Could you check a few things on this model? Use its own coordinates, in mm. A direction names the side the tool comes from. Round coordinates to 2 decimals unless told otherwise and drop trailing zeros. Loops run counter-clockwise (first coordinate to the right, second up) from the corner with the lowest first, then second, coordinate; pieces in that order, holes last. Notation, with made-up numbers: (10.5, 17.25) -> (17.5, 17.25) arc R23 cw to (17.5, 54.25) -> close; hole circle Ø8 at (74, 45.5). An arc over 180 degrees is marked (long way). One line per item, written item: value.
```python
from build123d import *

# Parameters (mm, degrees)
SKETCH1_R           = 28.575
SKETCH1_R_2         = 14.2875
SKETCH1_R_3         = 2.667
BOSS_EXTRUDE1_DEPTH = 6.35
BOSS_EXTRUDE2_DEPTH = 6.35
SKETCH3_W           = 25.4
SKETCH3_H           = 12.7
BOSS_EXTRUDE3_DEPTH = 6.35
CUT_EXTRUDE4_REACH  = 101.646
SKETCH4_R           = 4.7625
FILLET1_R           = 6.35
SKETCH5_W           = 86.18949407
SKETCH5_H           = 10.684979127
CUT_EXTRUDE5_DEPTH  = 100.646453148


with BuildPart() as part:
    # Sketch1 → Boss-Extrude1 (new body)
    with BuildSketch(Plane(origin=(0, 0, 0), x_dir=(1, 0, 0), z_dir=(0, 1, 0))):
        with Locations(Location((0, 0, 0), (0, 0, 270))):
            Circle(SKETCH1_R)
        with Locations(Location((0, 0, 0), (0, 0, 270))):
            Circle(SKETCH1_R_2, mode=Mode.SUBTRACT)
        with Locations(Location((11.90625, 20.622229928, 0), (0, 0, 270))):
            Circle(SKETCH1_R_3, mode=Mode.SUBTRACT)
        with Locations(Location((23.8125, 0, 0), (0, 0, 270))):
            Circle(SKETCH1_R_3, mode=Mode.SUBTRACT)
        with Locations(Location((11.90625, -20.622229928, 0), (0, 0, 270))):
            Circle(SKETCH1_R_3, mode=Mode.SUBTRACT)
        with Locations(Location((-11.90625, -20.622229928, 0), (0, 0, 270))):
            Circle(SKETCH1_R_3, mode=Mode.SUBTRACT)
        with Locations(Location((-23.8125, 0, 0), (0, 0, 270))):
            Circle(SKETCH1_R_3, mode=Mode.SUBTRACT)
        with Locations(Location((-11.90625, 20.622229928, 0), (0, 0, 270))):
            Circle(SKETCH1_R_3, mode=Mode.SUBTRACT)
    extrude(amount=BOSS_EXTRUDE1_DEPTH)

    # Sketch2 → Boss-Extrude2 (add)
    with BuildSketch(Plane(origin=(0, 0, 0), x_dir=(1, 0, 0), z_dir=(0, 1, 0))):
        with BuildLine():
            Line((26.940768363, -9.525), (95.25, -9.525))
            Line((95.25, -9.525), (95.25, 9.525))
            Line((95.25, 9.525), (26.940768363, 9.525))
            ThreePointArc((26.940768363, 9.525), (28.575, 0), (26.940768363, -9.525))
        make_face()
    extrude(amount=BOSS_EXTRUDE2_DEPTH)

    # Sketch3 → Boss-Extrude3 (add)
    with BuildSketch(Plane(origin=(0, 6.35, 0), x_dir=(1, 0, 0), z_dir=(0, 1, 0))):
        with Locations((82.55, 15.875)):
            Rectangle(SKETCH3_W, SKETCH3_H)
    extrude(amount=-BOSS_EXTRUDE3_DEPTH)

    # Sketch4 → Cut-Extrude4 (cut, up to next)
    with BuildSketch(Plane(origin=(0, 0, 0), x_dir=(1, 0, 0), z_dir=(0, 1, 0)), mode=Mode.PRIVATE) as cut_extrude4_sk1:
        with Locations(Location((82.55, 13.97, 0), (0, 0, 270))):
            Circle(SKETCH4_R)
    cut_extrude4_tool1 = extrude(cut_extrude4_sk1.sketch, amount=CUT_EXTRUDE4_REACH, mode=Mode.PRIVATE) & part.part
    add(cut_extrude4_tool1.solids().sort_by_distance((82.55, 0, -13.97))[0], mode=Mode.SUBTRACT)

    # Fillet1
    fillet1_edges = [part.edges().sort_by_distance(p)[0] for p in [
        (69.85, 3.175, -9.525),
        (95.25, 3.175, 9.525),
        (69.85, 3.175, -22.225),
        (95.25, 3.175, -22.225),
        (26.940768363, 3.175, 9.525),
        (26.940768363, 3.175, -9.525),
    ]]
    fillet(fillet1_edges, radius=FILLET1_R - 0.0001)  # a hair under: the kernel refuses the full size

    # Sketch5 → Cut-Extrude5 (cut, through all)
    with BuildSketch(Plane(origin=(0, 6.35, 0), x_dir=(1, 0, 0), z_dir=(0, 1, 0))):
        with Locations((4.822558491, 30.742489564)):
            Rectangle(SKETCH5_W, SKETCH5_H)
        with Locations((4.822558491, -30.742489564)):
            Rectangle(SKETCH5_W, SKETCH5_H)
    extrude(amount=-CUT_EXTRUDE5_DEPTH, mode=Mode.SUBTRACT)


solid = part.part
```
Item 1: If we section it at B-B on z = 0: Count the separate pieces of the cut face and the enclosed holes in it, plus the area to 3 significant figures.
Output:
separate pieces: 4
enclosed holes: 0
area: 537 mm²
Item 2: If we section it at A-A on x = 0: List the corners of the cut face in (y, z) for me, plus the area to 3 significant figures.
Output:
outline: (0, -25.4) -> (6.35, -25.4) -> (6.35, -14.29) -> (0, -14.29) -> close; (0, 14.29) -> (6.35, 14.29) -> (6.35, 25.4) -> (0, 25.4) -> close
area: 141 mm²
Item 3: If we section it at C-C on z = 11: List the corners of the cut face in (x, y) for me, plus the area to 3 significant figures.
Output:
outline: (-26.37, 0) -> (-9.12, 0) -> (-9.12, 6.35) -> (-26.37, 6.35) -> close; (9.12, 0) -> (27.04, 0) -> (27.04, 6.35) -> (9.12, 6.35) -> close
area: 223 mm²
Item 4: I need wall thicknesses on line 1 (X direction, y = 2, z = 18.5); line 2 (X direction, y = 2.5, z = -16); line 3 (Z direction, x = 82.55, y = 3.5) (1 decimal). Which ranges of each line are inside material? Lowest first, please. Write a range as from..to.
Output:
line 1: x = -21.78..-13.52, -10.29..10.29, 13.52..21.78
line 2: x = -23.68..23.68, 69.85..78.24, 86.86..95.25
line 3: z = -22.2..-18.7, -9.2..9.5
Item 5: If we mould it in two halves opening along Z, with no side actions, what happens to faces 4 (the face through (71.661, 3.131, -20.316)), 5 (the face through (32, 6.35, 0)), 6 (the face through (0, 3, 25.4)), 7 (the face through (-11.789, 3.131, 17.958))? For each: released by +Z, released by -Z, zero draft, split by the parting line, or undercut.
Output:
face 4: released by -Z
face 5: zero draft
face 6: released by +Z
face 7: undercut
Item 6: Will these pins go through, and if not, where does the flat tip stop? pin 1 Ø4 at (x, z) = (44.5, 9) entering from -Y; pin 2 Ø3 at (x, y) = (46, 4.5) entering from +Z (3 decimals); pin 3 Ø1 at (y, z) = (3.5, 12) entering from -X.
Output:
pin 1: stops at y = 0
pin 2: stops at z = 9.525
pin 3: stops at x = -26.16
Item 7: For faces 1 (the face through (82, 3, -22.225)), 2 (the face through (27.834, 3.219, -10.434)), 3 (the face through (93.439, 3.219, 7.616)), which set-ups out of +Z, -Z, +X, -X, +Y, -Y let a thin tool reach every point of the face, with its end or its side?
Output:
face 1: -Z, +X, +Y, -Y
face 2: -Z, +Y, -Y
face 3: +Z, +X, +Y, -Y
